Geometry: see drawing. Coordinates: mm, zero at the bounding-box minimum. A direction names the side the tool comes from. Give positions to 0.01 mm unless a question says otherwise; leave off trailing zeros. Loops run counter-clockwise (first coordinate to the right, second up) from the corner with the lowest first, then second, coordinate; pieces in that order, holes last. Notation, with made-up numbers: M -26.75,39.5 L 30.25,39.5 A21 ccw 30.25,68.5 Z; hole C 18,-22 d3. An arc over 180 degrees is marked long. Put each result on its own line as item: value.
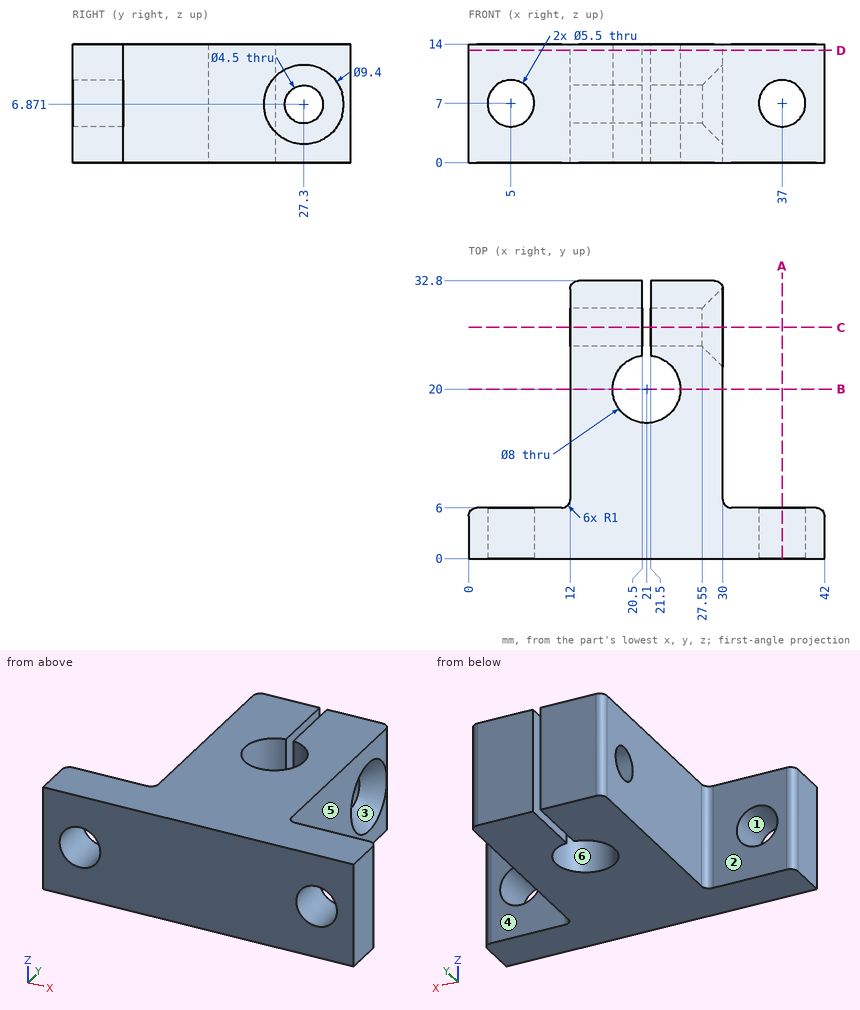
Item 1: Mould query, pull axis Y, two halves, no side actions, for the marked faces 3, 4, 5 and 6. Classes: pulls with the +Y half, pulls with the -Y half, needs draft (parallel to the pull), parting line crosses it, or undercut.
Output values:
face 3: undercut
face 4: pulls with the +Y half
face 5: needs draft
face 6: undercut
Item 2: Section C-C on y = 27.3. Output: boundary loops of the cut face in (x, z).
Output values:
outline: M 12,0 L 20.5,0 L 20.5,4.62 L 12,4.62 Z; M 12,9.12 L 20.5,9.12 L 20.5,14 L 12,14 Z; M 21.5,0 L 30,0 L 30,2.17 L 27.55,4.62 L 21.5,4.62 Z; M 21.5,9.12 L 27.55,9.12 L 30,11.57 L 30,14 L 21.5,14 Z
Item 3: Section D-D on z = 13.25. Output: boundary loops of the cut face in (x, y).
Output values:
outline: M 0,0 L 42,0 L 42,5 A1 ccw 41,6 L 31,6 A1 cw 30,7 L 30,31.8 A1 ccw 29,32.8 L 21.5,32.8 L 21.5,23.97 A4 cw long 20.5,23.97 L 20.5,32.8 L 13,32.8 A1 ccw 12,31.8 L 12,7 A1 cw 11,6 L 1,6 A1 ccw 0,5 Z
Item 4: Line query: probe 1 along X at (y, z) = (1.3, 7); probe 2 along Z at (x, y) = (26.25, 27.3); probe 3 along Y at (x, z) = (23, 7.75) (1 decimal). Output: solid intervals per line, ascending. Write a range as [from, to].
Output values:
probe 1: [0, 2.25], [7.75, 34.25], [39.75, 42]
probe 2: [0, 4.62], [9.12, 14]
probe 3: [0, 16.5], [23.5, 25.2], [29.4, 32.8]
Item 5: Section B-B on y = 20. Output: boundary loops of the cut face in (x, z), then the cut area to 3 significant figures.
Output values:
outline: M 12,0 L 17,0 L 17,14 L 12,14 Z; M 25,0 L 30,0 L 30,14 L 25,14 Z
area: 140 mm²
Item 6: Pin query (flat end, axial travel): pin 1 Ø4.5 at (y, z) = (27.5, 10) entering from +X; pin 2 Ø7 at (y, z) = (27.3, 6.87) entering from -X; pin 3 Ø5 at (y, z) = (27.3, 6.87) entering from +X; pin 4 Ø4.5 at (x, z) = (5, 7) entering from +Y. Return the tip coordinate at first contact, or that it passes through.
Output values:
pin 1: x = 30
pin 2: x = 12
pin 3: x = 27.8
pin 4: through
Item 7: Section A-A on x = 37. Output: boundary loops of the cut face in (y, z).
Output values:
outline: M 0,0 L 6,0 L 6,4.25 L 0,4.25 Z; M 0,9.75 L 6,9.75 L 6,14 L 0,14 Z
Item 8: Set-up query: the marked faces 1 and 2. Return all of +Z, -Z, +X, -X, +Y, -Y with unobstructed straight access to the full face (end or side cutting, diameter ignored); none if empty.
Output values:
face 1: +Y, -Y
face 2: +Z, -Z, -X, +Y
